Read the model definition and answer for the solid it produces. Units are mm, in the model's axes. Coordinates: 2 decimals unless noted, no trailing zeros. Write each loop counter-clockwise with the first axis right and the second up, starting at its lowest first coordinate (ties: lowest second). Pieces come first, ordered by that corner, then holes.
Item 1: Straight lines are drawn through the part: probe 1 along Z at (x, y) = (62.5, -19); probe 2 along Z at (x, y) = (-82.5, 37). For each, find the intervals that lie inside material, in ascending order.
Item 2: Section C-C (x = 69) is taken. Give the vertices of the cut face in (y, z).
Item 3: Section B-B (z = -4.5) is taken. Give the vertices of the cut face in (x, y), then the cut area to 3 significant figures.
Item 4: Section A-A (y = -6) is taken. Give the vertices of the cut face in (x, z), then the cut area to 3 significant figures.
from build123d import *

# Parameters (mm, degrees)
F1_DEPTH      = 57.15
F1_DEPTH_BACK = 57.15


with BuildPart() as f1:
    # F0 (on Front) → F1 (new body, two sides)
    with BuildSketch(Plane.XZ) as f1_sk:
        with BuildLine():
            Line((87.35775, 0), (-90.44225, 0))
            Line((-90.44225, 0), (-68.391527, -6.028698))
            ThreePointArc((-68.391527, -6.028698), (-66.731909, -6.365395), (-65.04225, -6.478296))
            Line((-65.04225, -6.478296), (61.95775, -6.478296))
            ThreePointArc((61.95775, -6.478296), (63.647409, -6.365395), (65.307026, -6.028698))
            Line((65.307026, -6.028698), (87.35775, 0))
        make_face()
    extrude(amount=F1_DEPTH)
    extrude(f1_sk.sketch, amount=-F1_DEPTH_BACK)


solid = f1.part
Established:
1. probe 1: z = -6.47 to 0
1. probe 2: z = -2.17 to 0
2. outline: (-57.15, -5.02) - (57.15, -5.02) - (57.15, 0) - (-57.15, 0) - close
3. outline: (-73.98, -57.15) - (70.9, -57.15) - (70.9, 57.15) - (-73.98, 57.15) - close
3. area: 16,600 mm2
4. outline: (-90.44, 0) - (-68.39, -6.03) arc R12.7 ccw to (-65.04, -6.48) - (61.96, -6.48) arc R12.7 ccw to (65.31, -6.03) - (87.36, 0) - close
4. area: 998 mm2
